Could you check a few things on this drawing? It's one solid part, dimensions in mm from its lowest x, y, z. A direction names the side the tool comes from. Round coordinates to 2 decimals unless told otherwise and drop trailing zeros. Write each loop counter-clockwise with the first axis right and the second up, starting at its lowest first coordinate (ties: lowest second). Pieces come first, ordered by that corner, then holes. Notation, with made-up numbers: (60, -34.5) - (118, -34.5) arc R14 cw to (118, -10.5) - close; hole circle Ø8 at (53, 38). An arc over 180 degrees is marked (long way). Write item = value, one per line. Start each with the question number.
Item 1: If we section it at A-A (x = 30): Please give me the cut outline in (y, z), and give its area (3 significant figures).
Item 2: Which directions (+Z, -Z, +X, -X, +Y, -Y) give clear straight access to the entire face, cutting with the end or side of a thin tool? Please do the marked faces 1 and 2.
Item 3: If we section it at C-C (z = 17): Please give me the cut outline in (x, y).
Item 4: If we section it at D-D (y = 35): Please give me the cut outline in (x, z).
Item 5: If I drill on line 1 along X through (y, z) = (27, 19.75); line 2 along Y through (x, z) = (13.5, 18.5); line 3 along Z through (x, y) = (35, 12), over which ranges is the centre line in solid material (lowest first)? Write a range as [from, to].
Item 6: If we section it at B-B (y = 10.5): Please give me the cut outline in (x, z).
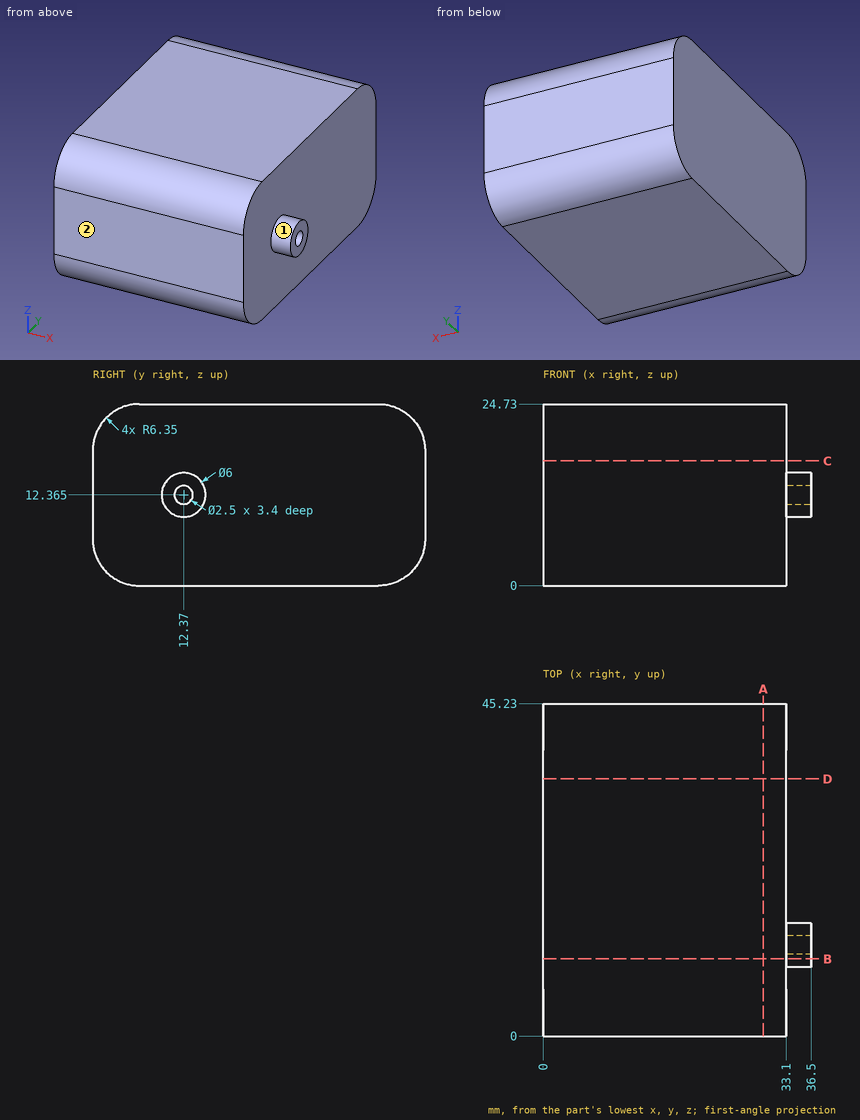
Reply:
q1.outline = (0, 6.35) arc R6.35 ccw to (6.35, 0) - (38.88, 0) arc R6.35 ccw to (45.23, 6.35) - (45.23, 18.38) arc R6.35 ccw to (38.88, 24.73) - (6.35, 24.73) arc R6.35 ccw to (0, 18.38) - close
q1.area = 1,080 mm2
q2.face_1 = +X
q2.face_2 = +Z, -Z, +X, -X, -Y
q3.outline = (0, 0) - (33.1, 0) - (33.1, 45.23) - (0, 45.23) - close
q4.outline = (0, 0) - (33.1, 0) - (33.1, 24.73) - (0, 24.73) - close
q5.line_1 = [0, 33.1]
q5.line_2 = [0, 45.23]
q5.line_3 = [9.39, 11.17], [13.56, 15.34]
q6.outline = (0, 0) - (33.1, 0) - (33.1, 10.02) - (36.5, 10.02) - (36.5, 14.71) - (33.1, 14.71) - (33.1, 24.73) - (0, 24.73) - close
